For this review, take the finished solid that the model builds, in its own axes (mm). A direction names the side the tool comes from. Coordinates: 2 decimals unless noted, no trailing zeros. Write each loop counter-clockwise with the first axis right and the second up, starting at its lowest first coordinate (ties: lowest second). Pieces come first, ordered by that corner, then holes. Notation, with made-up numbers: M -39.75,-7 L -22.75,-7 A16 ccw -22.75,2 Z; hole C 68,1.5 d1. An arc over 180 degrees is marked long. Return JSON: item names as keys, results as strings.
```python
from build123d import *

# Parameters (mm, degrees)
BOSS_EXTRUDE3_DEPTH             = 9.525
TAP_DRILL_FOR_M3X0_5_TAP1_D     = 2.5
TAP_DRILL_FOR_M3X0_5_TAP1_DEPTH = 9.895
M3_CLEARANCE_HOLE1_D            = 3.2
M3_CLEARANCE_HOLE2_D            = 3.2
M3_CLEARANCE_HOLE2_DEPTH        = 4.76
M3_CLEARANCE_HOLE2_TIP          = 0.96137699
M3_CLEARANCE_HOLE3_D            = 3.2
M3_CLEARANCE_HOLE3_DEPTH        = 9.895


with BuildPart() as part:
    # Sketch7 → Boss-Extrude3 (new body)
    with BuildSketch(Plane.XY):
        with BuildLine():
            Line((-11.8, 14.33255592), (-1.905, 14.33255592))
            Line((-1.905, 14.33255592), (-1.905, 9.33255592))
            ThreePointArc((-1.905, 9.33255592), (0, -9.525), (1.905, 9.33255592))
            Line((1.905, 9.33255592), (1.905, 14.33255592))
            Line((1.905, 14.33255592), (11.8, 14.33255592))
            Line((11.8, 14.33255592), (11.8, -12.96744408))
            Line((11.8, -12.96744408), (17.5, -12.96744408))
            Line((17.5, -12.96744408), (17.5, -17.73044408))
            Line((17.5, -17.73044408), (-17.5, -17.73044408))
            Line((-17.5, -17.73044408), (-17.5, -12.96744408))
            Line((-17.5, -12.96744408), (-11.8, -12.96744408))
            Line((-11.8, -12.96744408), (-11.8, 14.33255592))
        make_face()
    extrude(amount=BOSS_EXTRUDE3_DEPTH)

    # Tap Drill for M3x0.5 Tap1
    with Locations(Plane(origin=(11.8, 0, 0), x_dir=(0, 0, -1), z_dir=(1, 0, 0))):
        with Locations((-4.7625, 11.83255592)):
            Hole(TAP_DRILL_FOR_M3X0_5_TAP1_D / 2, depth=TAP_DRILL_FOR_M3X0_5_TAP1_DEPTH)

    # M3 Clearance Hole1 (through all)
    with Locations(Plane(origin=(0, -12.96744408, 0), x_dir=(1, 0, 0), z_dir=(0, 1, 0))):
        with Locations((-14.65, -4.749621695)):
            Hole(M3_CLEARANCE_HOLE1_D / 2)

    # M3 Clearance Hole2
    with Locations(Plane(origin=(0, -12.96744408, 0), x_dir=(1, 0, 0), z_dir=(0, 1, 0))):
        with Locations((14.65, -4.749621695)):
            Hole(M3_CLEARANCE_HOLE2_D / 2, depth=M3_CLEARANCE_HOLE2_DEPTH)
            with Locations((0, 0, -(M3_CLEARANCE_HOLE2_DEPTH + M3_CLEARANCE_HOLE2_TIP / 2))):  # 118° drill point
                Cone(0, M3_CLEARANCE_HOLE2_D / 2, M3_CLEARANCE_HOLE2_TIP, mode=Mode.SUBTRACT)

    # M3 Clearance Hole3
    with Locations(Plane.ZY.offset(11.8)):
        with Locations((4.7625, 11.83255592)):
            Hole(M3_CLEARANCE_HOLE3_D / 2, depth=M3_CLEARANCE_HOLE3_DEPTH)


solid = part.part
```
1. We need section A-A (y = 0). State the section outline as (x, z) points (3 decimals).
Checks:
{"outline": "M -11.8,0 L -9.525,0 L -9.525,9.525 L -11.8,9.525 Z; M 9.525,0 L 11.8,0 L 11.8,9.525 L 9.525,9.525 Z"}
2. We need section B-B (x = -8). State the section outline as (y, z) points (1 decimal).
Checks:
{"outline": "M -17.7,0 L -5.2,0 L -5.2,9.5 L -17.7,9.5 Z; M 5.2,0 L 14.3,0 L 14.3,9.5 L 5.2,9.5 Z; hole C 11.8,4.8 d3.2"}
3. We need section C-C (x = 14.65). State the section outline as (y, z) points (3 decimals).
Checks:
{"outline": "M -17.73,0 L -12.967,0 L -12.967,3.15 L -17.727,3.15 L -17.73,3.155 Z; M -17.73,6.345 L -17.727,6.35 L -12.967,6.35 L -12.967,9.525 L -17.73,9.525 Z"}
4. For faces 4 (the face through (1.905, 10.7, 3.6)), 5 (the face through (-6.783, 12.313, 3.236)), 6 (the face through (13, -12.967, 4)), 7 (the face through (-11.8, 0, 5)), list the 3-axis set-ups (+Z, -Z, +X, -X, +Y, -Y) from which the entire face can be reached by the end or side of a thin tool; tool diameter is ignored.
Checks:
{"face 4": "+Z, -Z, +Y", "face 5": "-X", "face 6": "+Z, -Z, +X, +Y", "face 7": "+Z, -Z, -X, +Y"}
5. Draft analysis for pull direction X (two halves, no side actions). For faces 1 (the face through (13.124, -15.381, 4.269)), 2 (the face through (-8, -9, 0)), 3 (the face through (11.8, 1, 5)), state which applies: +X half, -X half, draft (parallel to the pull), parting line (faces both ways), or undercut.
Checks:
{"face 1": "undercut", "face 2": "draft", "face 3": "+X half"}
6. Wall thickness on L1, parallel to Z at x = -14.65, y = -15.55 (3 decimals); L2, parallel to Y at x = -4, z = 6; L3, parallel to X at y = 0, z = 7 (3 decimals): over which ranges is each line inside the solid? List them lowest first. Write a range as from..to.
Checks:
{"L1": "0..3.15, 6.35..9.525", "L2": "-17.73..-8.64, 8.64..10.82, 12.85..14.33", "L3": "-11.8..-9.525, 9.525..11.8"}
7. Clearance check with flat-ended pins moving along their axes: pin 1 Ø1.9 at (x, z) = (-14.65, 4.75) entering from +Y; pin 2 Ø4 at (y, z) = (10.5, 6.5) entering from +X; pin 3 Ø3 at (x, z) = (15.5, 6.5) entering from +Y; pin 4 Ø5 at (y, z) = (7.5, 6.5) entering from -X. State where each tip first meets the part, or that it passes through.
Checks:
{"pin 1": "through", "pin 2": "x = 11.8", "pin 3": "y = -12.97", "pin 4": "x = -11.8"}
8. We need section D-D (y = -10). State the section outline as (x, z) points (3 decimals).
Checks:
{"outline": "M -11.8,0 L 11.8,0 L 11.8,9.525 L -11.8,9.525 Z"}
